from build123d import *

# Parameters (mm, degrees)
BOSS_EXTRUDE2_DEPTH      = 5
BOSS_EXTRUDE2_DEPTH_BACK = 5
SKETCH1_R                = 5


with BuildPart() as part:
    # Sketch1 → Boss-Extrude2 (new, two sides: drawn at the far end of the back side and taken through both)
    with BuildSketch(Plane(origin=(0, 0, 0), x_dir=(1, 0, 0), z_dir=(0, 1, 0)).offset(-BOSS_EXTRUDE2_DEPTH_BACK)):
        with BuildLine():
            Line((-30, 12.882308015), (-15, 12.882308015))
            Line((-15, 12.882308015), (-15, 7.882308015))
            ThreePointArc((-15, 7.882308015), (-12.071067812, 0.811240203), (-5, -2.117691985))
            Line((-5, -2.117691985), (5, -2.117691985))
            ThreePointArc((5, -2.117691985), (12.071067812, 0.811240203), (15, 7.882308015))
            Line((15, 7.882308015), (15, 12.882308015))
            Line((15, 12.882308015), (30, 12.882308015))
            ThreePointArc((30, 12.882308015), (33.535533906, 11.417841921), (35, 7.882308015))
            Line((35, 7.882308015), (35, -7.117691985))
            Line((35, -7.117691985), (15, -27.117691985))
            Line((15, -27.117691985), (-15, -27.117691985))
            Line((-15, -27.117691985), (-35, -7.117691985))
            Line((-35, -7.117691985), (-35, 7.882308015))
            ThreePointArc((-35, 7.882308015), (-33.535533906, 11.417841921), (-30, 12.882308015))
        make_face()
        with Locations(Location((-25, 0, 0), (0, 0, 270))):
            Circle(SKETCH1_R, mode=Mode.SUBTRACT)
        with Locations(Location((25, 0, 0), (0, 0, 90))):
            Circle(SKETCH1_R, mode=Mode.SUBTRACT)
    extrude(amount=BOSS_EXTRUDE2_DEPTH + BOSS_EXTRUDE2_DEPTH_BACK)


solid = part.part
Could you check a few things on this model? Use its own coordinates, in mm. A direction names the side the tool comes from. Give positions to 0.01 mm unless a question says otherwise; leave off trailing zeros. Order: outer loops, then holes, each group sorted by start corner. A loop starts at its lowest first (then second) coordinate and runs counter-clockwise, first axis right, second up.
1. Suppose I cut it at B-B (z = 0). List the corners of the cut face in (x, y) for me, plus the area to 3 significant figures.
2. Will these pins go through, and if not, where does the flat tip stop? P1, Ø2.5, axis at y = -2.5, z = -11.5, coming from the +X side; P2, Ø3, axis at x = 2, y = -1, coming from the -Z side; P3, Ø12, axis at x = 4, z = -5, coming from the -Y side; P4, Ø5, axis at y = 3, z = 18.5, coming from the +X side.
3. Suppose I cut it at A-A (y = -2.75). List the corners of the cut face in (x, z) for me.
4. I need wall thicknesses on L1, parallel to X at y = -1.75, z = 0; L2, parallel to X at y = 2.75, z = 4; L3, parallel to Z at x = 20.5, y = -2. Which ranges of each line are inside material? Lowest first, please.
5. Suppose I cut it at D-D (x = -3.5). List the corners of the cut face in (y, z) for me.
6. We'd pull the mould along Z, two halves only. Please class faces 3 (the flat face through (-35, 0, 0)), 4 (the cylindrical face through (-29.88, -0.07, -1.08)), 5 (the flat face through (0, 0, 27.118)): pulls with the +Z half, pulls with the -Z half, needs draft (parallel to the pull), parting line crosses it, or undercut.
7. For faces 1 (the flat face through (15, 0, -10)), 2 (the flat face through (35, 0, 0)), which set-ups out of +Z, -Z, +X, -X, +Y, -Y let a thin tool reach every point of the face, with its end or its side?
8. Suppose I cut it at C-C (x = 25). List the corners of the cut face in (y, z) for me.
Solved:
1. outline: (-35, -5) - (-30, -5) - (-30, 5) - (-35, 5) - close; (-20, -5) - (-11.15, -5) - (-11.15, 5) - (-20, 5) - close; (11.15, -5) - (20, -5) - (20, 5) - (11.15, 5) - close; (30, -5) - (35, -5) - (35, 5) - (30, 5) - close
1. area: 277 mm2
2. P1: stops at x = 34.4
2. P2: stops at z = 2.12
2. P3: passes through
2. P4: stops at x = 26.12
3. outline: (-35, -7.88) arc R5 ccw to (-30, -12.88) - (-15, -12.88) - (-15, -7.88) arc R10 cw to (-5, 2.12) - (5, 2.12) arc R10 cw to (15, -7.88) - (15, -12.88) - (30, -12.88) arc R5 ccw to (35, -7.88) - (35, 7.12) - (15, 27.12) - (-15, 27.12) - (-35, 7.12) - close; hole circle Ø10 at (-25, 0); hole circle Ø10 at (25, 0)
4. L1: x = -35 to -30, -20 to -11.15, 11.15 to 20, 30 to 35
4. L2: x = -35 to -28, -22 to 22, 28 to 35
4. L3: z = -12.88 to -2.18, 2.18 to 21.62
5. outline: (-5, 2.12) - (5, 2.12) - (5, 27.12) - (-5, 27.12) - close
6. face 3: needs draft
6. face 4: undercut
6. face 5: pulls with the +Z half
7. face 1: -Z, +Y, -Y
7. face 2: +Z, -Z, +X, +Y, -Y
8. outline: (-5, -12.88) - (5, -12.88) - (5, -5) - (-5, -5) - close; (-5, 5) - (5, 5) - (5, 17.12) - (-5, 17.12) - close
